from build123d import *

# Parameters (mm, degrees)
CROQUIS1_W              = 22.6
CROQUIS1_H              = 22.6
SALIENTE_EXTRUIR1_DEPTH = 25
CROQUIS2_R              = 5.1
CORTAR_EXTRUIR1_DEPTH   = 30.671198156
CROQUIS3_R              = 1.25
CORTAR_EXTRUIR2_DEPTH   = 30.671198156
CROQUIS4_W              = 20
CROQUIS4_H              = 20
CROQUIS4_W_2            = 17.6
CROQUIS4_H_2            = 17.6
CORTAR_EXTRUIR3_DEPTH   = 15
CROQUIS5_R              = 2.5
CORTAR_EXTRUIR4_DEPTH   = 36.545041848
CHAFL_N1_SIZE           = 2
REDONDEO1_R             = 2
REDONDEO2_R             = 2


with BuildPart() as part:
    # Croquis1 → Saliente-Extruir1 (new body)
    with BuildSketch(Plane.XY):
        Rectangle(CROQUIS1_W, CROQUIS1_H)
    extrude(amount=SALIENTE_EXTRUIR1_DEPTH)

    # Croquis2 → Cortar-Extruir1 (cut, through all)
    with BuildSketch(Plane.XY.offset(25)):
        Circle(CROQUIS2_R)
    extrude(amount=-CORTAR_EXTRUIR1_DEPTH, mode=Mode.SUBTRACT)

    # Croquis3 → Cortar-Extruir2 (cut, through all)
    with BuildSketch(Plane.XY.offset(25)):
        with Locations((5.656854249, 5.656854249)):
            Circle(CROQUIS3_R)
        with Locations((5.656854249, -5.656854249)):
            Circle(CROQUIS3_R)
        with Locations((-5.656854249, -5.656854249)):
            Circle(CROQUIS3_R)
        with Locations((-5.656854249, 5.656854249)):
            Circle(CROQUIS3_R)
    extrude(amount=-CORTAR_EXTRUIR2_DEPTH, mode=Mode.SUBTRACT)

    # Croquis4 → Cortar-Extruir3 (cut)
    with BuildSketch(Plane(origin=(0, 0, 0), x_dir=(-1, 0, 0), z_dir=(0, 0, -1))):
        Rectangle(CROQUIS4_W, CROQUIS4_H)
        Rectangle(CROQUIS4_W_2, CROQUIS4_H_2, mode=Mode.SUBTRACT)
    extrude(amount=-CORTAR_EXTRUIR3_DEPTH, mode=Mode.SUBTRACT)

    # Croquis5 → Cortar-Extruir4 (cut, through all)
    with BuildSketch(Plane(origin=(11.3, 0, 0), x_dir=(0, 0, -1), z_dir=(1, 0, 0))):
        with Locations(Location((-9, 0, 0), (0, 0, 90))):
            Circle(CROQUIS5_R)
    extrude(amount=-CORTAR_EXTRUIR4_DEPTH, mode=Mode.SUBTRACT)

    # Chaflán1
    # the kernel refuses this chamfer: 2 mm, written as the material it takes off along each edge
    with BuildSketch(Plane(origin=(-11.3, 0, 9), x_dir=(0, 1, 0), z_dir=(0, 0, -1))) as chafl_n1_piece_1:
        Polygon((2.5 + CHAFL_N1_SIZE, 0), (2.5, CHAFL_N1_SIZE), (2.5, 0), align=None)
    revolve(axis=Axis((-11.3, 0, 9), (1, 0, 0)), mode=Mode.SUBTRACT)
    with BuildSketch(Plane(origin=(11.3, 0, 9), x_dir=(0, 1, 0), z_dir=(0, 0, -1))) as chafl_n1_piece_2:
        Polygon((2.5 + CHAFL_N1_SIZE, 0), (2.5, -CHAFL_N1_SIZE), (2.5, 0), align=None)
    revolve(axis=Axis((11.3, 0, 9), (1, 0, 0)), mode=Mode.SUBTRACT)

    # Redondeo1
    redondeo1_edges = [part.edges().sort_by_distance(p)[0] for p in [
        (11.3, -11.3, 12.5),
        (-11.3, -11.3, 12.5),
        (-11.3, 11.3, 12.5),
        (11.3, 11.3, 12.5),
    ]]
    fillet(redondeo1_edges, radius=REDONDEO1_R)

    # Redondeo2
    redondeo2_edges = [part.edges().sort_by_distance(p)[0] for p in [
        (0, -11.3, 25),
        (-11.3, 0, 25),
        (11.3, 0, 25),
        (0, 11.3, 25),
        (10.714213562, 10.714213562, 25),
        (-10.714213562, 10.714213562, 25),
        (10.714213562, -10.714213562, 25),
        (-10.714213562, -10.714213562, 25),
    ]]
    fillet(redondeo2_edges, radius=REDONDEO2_R)


solid = part.part
Read the model definition and answer for the solid it produces. Units are mm, in the model's axes. A direction names the side the tool comes from. Coordinates: 2 decimals unless noted, no trailing zeros. Loops run counter-clockwise (first coordinate to the right, second up) from the corner with the lowest first, then second, coordinate; pieces in that order, holes last. Notation, with made-up numbers: (84, 62.25) -> (102, 62.25) arc R29 cw to (102, 101.25) -> close; hole circle Ø9 at (-22.5, 35.25). An arc over 180 degrees is marked (long way). Write item = value, one per line. Start each with the question number.
1) The mould has two halves that part along Y. Classify faces 1 (the face through (10.7, 10.73, 11.66)), 2 (the face through (-4, -4, 25)), 3 (the face through (10, 2, 6)), 4 (the face through (-8.8, 0, 6)): pulls with the +Y half, pulls with the -Y half, needs draft (parallel to the pull), parting line crosses it, or undercut.
2) Find the intervals of material crossed by L1, parallel to Y at x = 0, z = 13.75; L2, parallel to X at y = 9, z = 1.5, in increasing order. Write a range as from..to.
3) The part is cut by section A-A, the plane x = 0. Determine the outline of the cut face in (y, z).
4) The part is cut by section B-B, the plane y = 0. State how many separate pieces and enclosed holes the cut face has, plus the area to 3 significant figures.
5) For faces 5 (the face through (0, -11.3, 11)), 6 (the face through (0, 8.8, 7)), determine the directions among +Z, -Z, +X, -X, +Y, -Y from which every point of the face is accessible in a straight line to the end or side of a thin tool.
6) Given P1, Ø2, axis at x = -5.66, y = -5.66, coming from the -Z side; P2, Ø12, axis at y = 2.5, z = 9.5, coming from the +X side, each flat-ended and moving along its own axis, determine where each tip first touches the part or whether it passes through.
7) The part is cut by section D-D, the plane x = -5.5. Determine the outline of the cut face in (y, z), plus the area to 3 significant figures.
8) The part is cut by section C-C, the plane z = 3.25. Determine the outline of the cut face in (x, y).
Result:
q1.face_1 = pulls with the +Y half
q1.face_2 = needs draft
q1.face_3 = undercut
q1.face_4 = undercut
q2.L1 = -11.3..-10, -8.8..-5.1, 5.1..8.8, 10..11.3
q2.L2 = -11.3..-10, 10..11.3
q3.outline = (-11.3, 0) -> (-10, 0) -> (-10, 15) -> (-8.8, 15) -> (-8.8, 0) -> (-5.1, 0) -> (-5.1, 25) -> (-9.3, 25) arc R2 ccw to (-11.3, 23) -> close; (5.1, 0) -> (8.8, 0) -> (8.8, 15) -> (10, 15) -> (10, 0) -> (11.3, 0) -> (11.3, 23) arc R2 ccw to (9.3, 25) -> (5.1, 25) -> close
q4.separate_pieces = 6
q4.enclosed_holes = 0
q4.area = 215 mm²
q5.face_5 = +Z, -Z, +X, -X, -Y
q5.face_6 = -Z
q6.P1 = through
q6.P2 = 11.3
q7.outline = (-11.3, 0) -> (-10, 0) -> (-10, 15) -> (-8.8, 15) -> (-8.8, 0) -> (-6.9, 0) -> (-6.9, 25) -> (-9.3, 25) arc R2 ccw to (-11.3, 23) -> close; (-4.42, 0) -> (4.42, 0) -> (4.42, 25) -> (-4.42, 25) -> close; (6.9, 0) -> (8.8, 0) -> (8.8, 15) -> (10, 15) -> (10, 0) -> (11.3, 0) -> (11.3, 23) arc R2 ccw to (9.3, 25) -> (6.9, 25) -> close; hole circle Ø5 at (0, 9)
q7.area = 384 mm²
q8.outline = (-11.3, -9.3) arc R2 ccw to (-9.3, -11.3) -> (9.3, -11.3) arc R2 ccw to (11.3, -9.3) -> (11.3, 9.3) arc R2 ccw to (9.3, 11.3) -> (-9.3, 11.3) arc R2 ccw to (-11.3, 9.3) -> close; (-8.8, -8.8) -> (8.8, -8.8) -> (8.8, 8.8) -> (-8.8, 8.8) -> close; hole (-10, -10) -> (10, -10) -> (10, 10) -> (-10, 10) -> close; hole circle Ø2.5 at (-5.66, -5.66); hole circle Ø2.5 at (-5.66, 5.66); hole circle Ø10.2 at (0, 0); hole circle Ø2.5 at (5.66, -5.66); hole circle Ø2.5 at (5.66, 5.66)
